Here's how the part is built. I have some questions about the finished solid (model axes, mm). Give positions to 0.01 mm unless a question says otherwise; leave off trailing zeros. Write each loop counter-clockwise with the first axis right and the second up, starting at its lowest first coordinate (ties: lowest second). Pieces come first, ordered by that corner, then holes. Notation, with made-up numbers: (-32, 2.5) -> (-14, 2.5) arc R20 ccw to (-14, 22.5) -> close; hole circle Ø6 at (-8.75, 37.25). An arc over 180 degrees is marked (long way). Answer as CSV lines item,"result". Start each with the question number.
from build123d import *

# Parameters (mm, degrees)
CROQUIS1_W                 = 73.8
CROQUIS1_H                 = 73.8
SALIENTE_EXTRUIR3_DEPTH    = 1.9
CROQUIS2_R                 = 2.5
CORTAR_EXTRUIR1_DEPTH      = 1
CORTAR_EXTRUIR1_DEPTH_BACK = 2.9


with BuildPart() as part:
    # Croquis1 → Saliente-Extruir3 (new body)
    with BuildSketch(Plane(origin=(0, 0, 0), x_dir=(1, 0, 0), z_dir=(0, 1, 0))):
        Rectangle(CROQUIS1_W, CROQUIS1_H)
    extrude(amount=SALIENTE_EXTRUIR3_DEPTH)

    # Croquis2 → Cortar-Extruir1 (cut, two sides)
    with BuildSketch(Plane(origin=(0, 1.9, 0), x_dir=(1, 0, 0), z_dir=(0, 1, 0))) as cortar_extruir1_sk:
        with Locations((-27, 0)):
            Circle(CROQUIS2_R)
        with Locations((27, 0)):
            Circle(CROQUIS2_R)
    extrude(amount=CORTAR_EXTRUIR1_DEPTH, mode=Mode.SUBTRACT)
    extrude(cortar_extruir1_sk.sketch, amount=-CORTAR_EXTRUIR1_DEPTH_BACK, mode=Mode.SUBTRACT)


solid = part.part
Item 1: If we section it at A-A (x = 27): Please give me the cut outline in (y, z), and give its area (3 significant figures).
Item 2: If we section it at B-B (z = 0): Please give me the cut outline in (x, y), and give its area (3 significant figures).
Item 3: If I drill on line 1 (X direction, y = 0.9, z = 0); line 2 (Z direction, x = -27, y = 1.15); line 3 (X direction, y = 0.9, z = 1.5), over which ranges is the centre line in solid material (lowest first)? Write a range as [from, to].
Item 4: If we section it at C-C (x = -28.5): Please give me the cut outline in (y, z), and give its area (3 significant figures).
Item 5: I'm going to push flat-ended pins straight in: pin 1 (6 mm diameter, centred on x = 27, z = 0, fed in from +Y); pin 2 (4 mm diameter, centred on x = -27, z = 0, fed in from +Y). Where does each tip first touch, or does it pass through?
Item 6: We'd pull the mould along X, two halves only. Please class faces 1 (the face through (-1, 1.9, -1)), 2 (the face through (-29.5, 1, -0.1)), 3 (the face through (-36.9, 1, 1)): released by +X, released by -X, zero draft, split by the parting line, or undercut.
Final values:
1,outline,"(0, -36.9) -> (1.9, -36.9) -> (1.9, -2.5) -> (0, -2.5) -> close; (0, 2.5) -> (1.9, 2.5) -> (1.9, 36.9) -> (0, 36.9) -> close"
1,area,"131 mm2"
2,outline,"(-36.9, 0) -> (-29.5, 0) -> (-29.5, 1.9) -> (-36.9, 1.9) -> close; (-24.5, 0) -> (24.5, 0) -> (24.5, 1.9) -> (-24.5, 1.9) -> close; (29.5, 0) -> (36.9, 0) -> (36.9, 1.9) -> (29.5, 1.9) -> close"
2,area,"121 mm2"
3,line 1,"[-36.9, -29.5], [-24.5, 24.5], [29.5, 36.9]"
3,line 2,"[-36.9, -2.5], [2.5, 36.9]"
3,line 3,"[-36.9, -29], [-25, 25], [29, 36.9]"
4,outline,"(0, -36.9) -> (1.9, -36.9) -> (1.9, -2) -> (0, -2) -> close; (0, 2) -> (1.9, 2) -> (1.9, 36.9) -> (0, 36.9) -> close"
4,area,"133 mm2"
5,pin 1,"y = 1.9"
5,pin 2,"through"
6,face 1,"zero draft"
6,face 2,"undercut"
6,face 3,"released by -X"
